Could you check a few things on this model? Use its own coordinates, in mm. Face numbers are marked on the shaded views. A direction names the side the tool comes from. Round coordinates to 2 decimals unless told otherwise and drop trailing zeros. Order: outer loops, then holes, each group sorted by start corner. A loop starts at its lowest first (then second) coordinate and runs counter-clockwise, first axis right, second up.
```python
from build123d import *

# Parameters (mm, degrees)
F1_DEPTH = 90
F0_W     = 10
F0_H     = 1
F2_DEPTH = 39
F0_W_2   = 20
F3_DEPTH = 25
F4_DEPTH = 1
F5_R     = 5
F6_R     = 5
F7_R     = 5
F8_R     = 5


with BuildPart() as f1:
    # F0 (on Top) → F1 (new body)
    with BuildSketch(Plane.XY):
        with BuildLine():
            ThreePointArc((58.273254, 16.21197), (39.155261, 45.99313), (5.273254, 56.21197))
            Line((5.273254, 56.21197), (5.273254, 55.117212))
            ThreePointArc((5.273254, 55.117212), (38.296792, 45.052118), (57.273254, 16.21197))
            Line((57.273254, 16.21197), (58.273254, 16.21197))
        make_face()
        Polygon((5.273254, 16.21197), (5.273254, 15.21197), (57.273254, 15.21197), (58.273254, 15.21197), (58.273254, 16.21197), (57.273254, 16.21197), align=None)
        Polygon((4.273254, 56.21197), (4.273254, 55.21197), (4.273254, 15.21197), (5.273254, 15.21197), (5.273254, 16.21197), (5.273254, 55.117212), (5.273254, 56.21197), align=None)
    extrude(amount=F1_DEPTH)

    # F0 (on Top) → F2 (join)
    with BuildSketch(Plane.XY):
        Polygon((58.273254, 15.21197), (57.273254, 15.21197), (57.273254, -36.78803), (47.273254, -36.78803), (47.273254, -37.78803), (58.273254, -37.78803), align=None)
        Polygon((5.273254, 15.21197), (4.273254, 15.21197), (4.273254, -36.78803), (4.273254, -37.78803), (5.273254, -37.78803), (5.273254, -36.78803), align=None)
        with Locations((10.273254, -37.28803)):
            Rectangle(F0_W, F0_H)
    extrude(amount=F2_DEPTH)

    # F0 (on Top) → F3 (join)
    with BuildSketch(Plane.XY):
        Polygon((-87.726746, -36.78803), (-87.726746, 55.21197), (4.273254, 55.21197), (4.273254, 56.21197), (-88.726746, 56.21197), (-88.726746, -37.78803), (-67.726746, -37.78803), (-67.726746, -36.78803), align=None)
        with Locations((-5.726746, -37.28803)):
            Rectangle(F0_W_2, F0_H)
    extrude(amount=F3_DEPTH)

    # F0 (on Top) → F4 (join)
    with BuildSketch(Plane.XY):
        Polygon((4.273254, 55.21197), (-87.726746, 55.21197), (-87.726746, -36.78803), (-67.726746, -36.78803), (-15.726746, -36.78803), (4.273254, -36.78803), (4.273254, 15.21197), align=None)
        Polygon((57.273254, 15.21197), (5.273254, 15.21197), (5.273254, -36.78803), (15.273254, -36.78803), (47.273254, -36.78803), (57.273254, -36.78803), align=None)
        with BuildLine():
            Line((5.273254, 55.117212), (5.273254, 16.21197))
            Line((5.273254, 16.21197), (57.273254, 16.21197))
            ThreePointArc((57.273254, 16.21197), (38.296792, 45.052118), (5.273254, 55.117212))
        make_face()
    extrude(amount=F4_DEPTH)

    # F5
    f5_edges = [f1.edges().sort_by_distance(p)[0] for p in [
        (-67.726746, -37.28803, 25),
    ]]
    fillet(f5_edges, radius=F5_R)

    # F6
    f6_edges = [f1.edges().sort_by_distance(p)[0] for p in [
        (-15.726746, -37.28803, 25),
    ]]
    fillet(f6_edges, radius=F6_R)

    # F7
    f7_edges = [f1.edges().sort_by_distance(p)[0] for p in [
        (15.273254, -37.28803, 39),
    ]]
    fillet(f7_edges, radius=F7_R)

    # F8
    f8_edges = [f1.edges().sort_by_distance(p)[0] for p in [
        (47.273254, -37.28803, 39),
    ]]
    fillet(f8_edges, radius=F8_R)


solid = f1.part
```
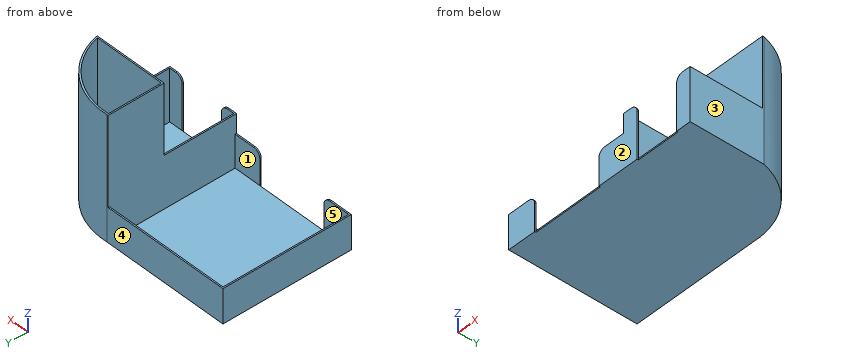
Q1. For the marked faces 1 and 2, which set-ups out of +Z, -Z, +X, -X, +Y, -Y let a thin tool reach every point of the face, with its end or its side?
Q2. I need wall thicknesses on L1, parallel to X at y = 23, z = 20.5; L2, parallel to Y at x = -78, z = 12; L3, parallel to X at y = 23, z = 84. Which ranges of each line are inside material? Lowest first, please.
Q3. We'd pull the mould along X, two halves only. Please class the marked faces 3, 4 and 5: released by +X, released by -X, zero draft, split by the parting line, or undercut.
Q4. Imagine slicing it at D-D, the plane z = 31.5. Please give me the cut outline in (x, y), then the cut area to 3 significant figures.
Q5. Imagine slicing it at C-C, the plane x = 29.5. Please give me the cut outline in (y, z), then the cut area to 3 significant figures.
Q6. Imagine slicing it at A-A, the plane z = 17.5. Please give me the cut outline in (x, y).
Q7. Imagine slicing it at B-B, the plane y = 6.5. Please give me the cut outline in (x, z), then the cut area to 3 significant figures.
Q8. For P1, Ø1, axis at x = 41.5, z = 54.5, coming from the -Y side; P2, Ø6, axis at y = 10.5, z = 33, coming from the -X side; P3, Ø16, axis at x = 43.5, z = 29, coming from the -Y side; P4, Ø6, axis at x = -63, y = 31, coming from the +Z side, each with a flat end and sliding along its axis, tell me the tip position at first contact or that it passes through.
Filled in:
1. face 1: +Z
1. face 2: +Z, -Z, +X, -X, -Y
2. L1: x = -88.73 to -87.73, 4.27 to 5.27, 55.13 to 56.27
2. L2: y = -37.79 to -36.79, 55.21 to 56.21
2. L3: x = 4.27 to 5.27, 55.13 to 56.27
3. face 3: released by +X
3. face 4: zero draft
3. face 5: undercut
4. outline: (4.27, -37.79) - (15.27, -37.79) - (15.27, -36.79) - (5.27, -36.79) - (5.27, 15.21) - (57.27, 15.21) - (57.27, -36.79) - (47.27, -36.79) - (47.27, -37.79) - (58.27, -37.79) - (58.27, 16.21) arc R51.1 ccw to (5.27, 56.21) - (4.27, 56.21) - close; hole (5.27, 16.21) - (57.27, 16.21) arc R50.83 ccw to (5.27, 55.12) - close
4. area: 305 mm2
5. outline: (-36.79, 0) - (51.73, 0) - (51.73, 90) - (50.34, 90) - (50.34, 1) - (16.21, 1) - (16.21, 90) - (15.21, 90) - (15.21, 1) - (-36.79, 1) - close
5. area: 302 mm2
6. outline: (-88.73, -37.79) - (-67.73, -37.79) - (-67.73, -36.79) - (-87.73, -36.79) - (-87.73, 55.21) - (4.27, 55.21) - (4.27, -36.79) - (-15.73, -36.79) - (-15.73, -37.79) - (15.27, -37.79) - (15.27, -36.79) - (5.27, -36.79) - (5.27, 15.21) - (57.27, 15.21) - (57.27, -36.79) - (47.27, -36.79) - (47.27, -37.79) - (58.27, -37.79) - (58.27, 16.21) arc R51.1 ccw to (5.27, 56.21) - (-88.73, 56.21) - close; hole (5.27, 16.21) - (57.27, 16.21) arc R50.83 ccw to (5.27, 55.12) - close
7. outline: (-88.73, 0) - (58.27, 0) - (58.27, 39) - (57.27, 39) - (57.27, 1) - (5.27, 1) - (5.27, 39) - (4.27, 39) - (4.27, 1) - (-87.73, 1) - (-87.73, 25) - (-88.73, 25) - close
7. area: 247 mm2
8. P1: stops at y = 15.21
8. P2: stops at x = 4.27
8. P3: stops at y = -37.79
8. P4: stops at z = 1
